```python
from build123d import *

# Parameters (mm, degrees)
F0_R            = 150
F1_DEPTH        = 2.5
F2_R            = 29
F3_DEPTH        = 5.001
F3_COPIES_COUNT = 8
F2_R_2          = 30
F4_DEPTH        = 2
F4_COPIES_COUNT = 8
F5_R            = 2.0850492766
F6_DEPTH        = 5.001


# Not quite as in the source:
# - a pattern or mirror of a feature is missing from the dataset's text; its kind, count and spacing are read off the source's solid


with BuildPart() as f1:
    # F0 (on Top) → F1 (new body, symmetric)
    with BuildSketch(Plane.XY):
        Circle(F0_R)
    extrude(amount=F1_DEPTH, both=True)

    # F2 (on face) → F3 (cut, through all)
    with BuildSketch(Plane.XY.offset(2.5)):
        with Locations((17.6781384332, 105.6203827018)):
            Circle(F2_R)
    f3 = extrude(amount=-F3_DEPTH, mode=Mode.SUBTRACT)

    # F3_copies: F3 ×8 about axis
    f3_copies_axis = Axis((0, 0, 0), (0, 0, 1))
    for i in range(1, F3_COPIES_COUNT):
        add(f3.rotate(f3_copies_axis, i * 360 / F3_COPIES_COUNT), mode=Mode.SUBTRACT)

    # F2 (on face) → F4 (cut)
    with BuildSketch(Plane.XY.offset(2.5)):
        with Locations((17.6781384332, 105.6203827018)):
            Circle(F2_R_2)
        with Locations((17.6781384332, 105.6203827018)):
            Circle(F2_R, mode=Mode.SUBTRACT)
    f4 = extrude(amount=-F4_DEPTH, mode=Mode.SUBTRACT)

    # F4_copies: F4 ×8 about axis
    f4_copies_axis = Axis((0, 0, 0), (0, 0, 1))
    for i in range(1, F4_COPIES_COUNT):
        add(f4.rotate(f4_copies_axis, i * 360 / F4_COPIES_COUNT), mode=Mode.SUBTRACT)

    # F5 (on face) → F6 (cut, through all)
    with BuildSketch(Plane.XY.offset(2.5)):
        with Locations((84.5384001732, -116.1978319287)):
            Circle(F5_R)
    extrude(amount=-F6_DEPTH, mode=Mode.SUBTRACT)


solid = f1.part
```
Input: part model. Units: mm. Frame: model coordinates. A direction names the side the tool comes from. Round coordinates to 2 decimals unless told otherwise and drop trailing zeros. Write each loop counter-clockwise with the first axis right and the second up, starting at its lowest first coordinate (ties: lowest second). Pieces come first, ordered by that corner, then holes. Notation, with made-up numbers: (82, -0.75) - (98, -0.75) arc R18 ccw to (98, 16.25) - close; hole circle Ø8 at (81, 45.25). An arc over 180 degrees is marked (long way). Write item = value, one per line.
(1) Material intervals for probe 1 along Y at (x, z) = (-61.5, -0.25); probe 2 along Y at (x, z) = (37, -1.9); probe 3 along Y at (x, z) = (-88, 1.6), sorted ascending.
Geometry check:
probe_1 = -136.81 to -75.65, -48.72 to 58.19, 116.18 to 136.81
probe_2 = -145.37 to -101.56, -72.81 to 83.99, 127.25 to 145.37
probe_3 = -121.47 to -92.17, -32.2 to -6.6, 41.96 to 71.9, 102.47 to 121.47
(2) Section query B-B on y = -18.5. Output: boundary loops of the cut face in (x, z).
Geometry check:
outline = (-148.85, -2.5) - (76.63, -2.5) - (76.63, 0.5) - (75.63, 0.5) - (75.63, 2.5) - (-148.85, 2.5) - close; (134.61, -2.5) - (148.85, -2.5) - (148.85, 2.5) - (135.61, 2.5) - (135.61, 0.5) - (134.61, 0.5) - close
(3) Section query D-D on x = -17. Output: boundary loops of the cut face in (y, z), then the cut area to 3 significant figures.
Geometry check:
outline = (-149.03, -2.5) - (-134.61, -2.5) - (-134.61, 0.5) - (-135.61, 0.5) - (-135.61, 2.5) - (-149.03, 2.5) - close; (-76.63, -2.5) - (149.03, -2.5) - (149.03, 2.5) - (-75.63, 2.5) - (-75.63, 0.5) - (-76.63, 0.5) - close
area = 1,200 mm^2
(4) Section query C-C on z = -1.5. State how many separate pieces and enclosed holes the cut face has, then the cut area to 3 significant figures.
Geometry check:
separate_pieces = 1
enclosed_holes = 9
area = 49,500 mm^2
(5) Access query for faces 1 (the cylindrical face through (125.9, 4.43, 1.51)), 2 (the cylindrical face through (67.6, 83.57, -0.98)). Directions: +Z, -Z, +X, -X, +Y, -Y. A direction counts if a zero-diameter tool reaches every point of the face in a straight line with its end or side. Return the directions, or none.
Geometry check:
face_1 = +Z
face_2 = +Z, -Z
(6) Pull-direction query (Y, two-part tool) for faces 3 (the flat face through (-2, 2, -2.5)), 4 (the flat face through (81, 91, 0.5)); classes: +Y half, -Y half, draft (parallel to the pull), parting line (faces both ways), or undercut.
Geometry check:
face_3 = draft
face_4 = undercut
(7) Section query A-A on x = 102. Output: boundary loops of the cut face in (y, z), then the cut area to 3 significant figures.
Geometry check:
outline = (-109.98, -2.5) - (-46.45, -2.5) - (-46.45, 0.5) - (-47.46, 0.5) - (-47.46, 2.5) - (-109.98, 2.5) - close; (11.09, -2.5) - (37.25, -2.5) - (37.25, 0.5) - (36.1, 0.5) - (36.1, 2.5) - (12.1, 2.5) - (12.1, 0.5) - (11.09, 0.5) - close; (87.11, -2.5) - (109.98, -2.5) - (109.98, 2.5) - (88.27, 2.5) - (88.27, 0.5) - (87.11, 0.5) - close
area = 554 mm^2
(8) Contact query for a flat-ended pin moving along its axis: pin 1 Ø1 at (x, z) = (-52.5, 0) entering from +Y. Output: stop coordinate, or through.
Geometry check:
pin_1 = 140.7
